Geometry check sheet. Reference: the model listing, model coordinates, mm. A direction names the side the tool comes from. Give positions to 0.01 mm unless a question says otherwise; leave off trailing zeros. Loops run counter-clockwise (first coordinate to the right, second up) from the corner with the lowest first, then second, coordinate; pieces in that order, holes last. Notation, with made-up numbers: (-32.75, -12.5) - (-15.75, -12.5) arc R22 cw to (-15.75, 3.5) - close; hole circle Ø3 at (-36, 86). An arc over 180 degrees is marked (long way). Use a Markdown table: item, result. Add a question column.
1. Cross-section at A-A on y = 3.75. Enter the section's corners in (x, z), and give its area (3 significant figures).
2. Draft check along Z on faces 4 (the flat face through (1, 5, 15.347)), 5 (the cylindrical face through (4.436, 12.686, 14.995)), 6 (the cylindrical face through (-16.435, 0.783, -11.827)), 7 (the flat face through (-18, 7, -4.453)). Enter one of: pulls with the +Z half, pulls with the -Z half, needs draft (parallel to the pull), parting line crosses it, or undercut.
3. Set-up check for faces 1 (the flat face through (-3.366, 7, 13)), 2 (the flat face through (6.134, 7, 13)), 3 (the flat face through (18, 7, -3.348)): record each of +Z, -Z, +X, -X, +Y, -Y from which the full face is reachable in a straight line by a thin tool's end or side.
4. Cross-section at B-B on z = 4. Enter the section's corners in (x, y), and give its area (3 significant figures).
5. Depth check by flat-ended pin: P1, Ø6, axis at y = 4.5, z = 12, coming from the +X side; P2, Ø3.5, axis at y = 8, z = 12.5, coming from the +X side; P3, Ø3.5, axis at y = 4.5, z = 12.5, coming from the -X side; P4, Ø10, axis at x = 1.5, z = 4.5, coming from the +Y side. Enter the tip coordinate at first touch or a pass-through.
6. Material ranges on L1, parallel to X at y = 4.5, z = 4.5; L2, parallel to Y at x = 0.5, z = 0; L3, parallel to Z at x = -15.5, y = 10, recorded low to high.
7. Cross-section at D-D on z = -12.5. Enter the section's corners in (x, y), and give its area (3 significant figures).
8. Cross-section at C-C on x = -18.5. Enter the section's corners in (y, z), and give its area (3 significant figures).
from build123d import *

# Parameters (mm, degrees)
SKETCH1_R           = 1.5875
BOSS_EXTRUDE4_DEPTH = 1.5875
SKETCH2_W           = 7.5057
SKETCH2_H           = 9.9695
BOSS_EXTRUDE5_DEPTH = 10.0711
SKETCH3_W           = 9.4996
SKETCH3_H           = 4.3434
BOSS_EXTRUDE6_DEPTH = 10.0965
SKETCH5_R           = 1.1303
BOSS_EXTRUDE7_DEPTH = 2.032
SKETCH6_W           = 7.5438
SKETCH6_H           = 9.9822
BOSS_EXTRUDE8_DEPTH = 11.1125


with BuildPart() as part:
    # Sketch1 → Boss-Extrude4 (new body)
    with BuildSketch(Plane(origin=(0, 0, 0), x_dir=(1, 0, 0), z_dir=(0, 1, 0))):
        with BuildLine():
            Line((21.881838929, -14.076705181), (21.881838929, 13.888694819))
            ThreePointArc((21.881838929, 13.888694819), (21.509864541, 14.786720431), (20.611838929, 15.158694819))
            Line((20.611838929, 15.158694819), (-20.612361071, 15.158694819))
            ThreePointArc((-20.612361071, 15.158694819), (-21.510386683, 14.786720431), (-21.882361071, 13.888694819))
            Line((-21.882361071, 13.888694819), (-21.882361071, -14.076705181))
            ThreePointArc((-21.882361071, -14.076705181), (-21.510386683, -14.974730793), (-20.612361071, -15.346705181))
            Line((-20.612361071, -15.346705181), (20.611838929, -15.346705181))
            ThreePointArc((20.611838929, -15.346705181), (21.509864541, -14.974730793), (21.881838929, -14.076705181))
        make_face()
        with Locations(Location((18.0086, 11.6205, 0), (0, 0, 270))):
            Circle(SKETCH1_R, mode=Mode.SUBTRACT)
        with Locations(Location((-18.0086, 11.6205, 0), (0, 0, 270))):
            Circle(SKETCH1_R, mode=Mode.SUBTRACT)
        with Locations(Location((-18.0086, -11.6205, 0), (0, 0, 270))):
            Circle(SKETCH1_R, mode=Mode.SUBTRACT)
        with Locations(Location((18.0086, -11.6205, 0), (0, 0, 270))):
            Circle(SKETCH1_R, mode=Mode.SUBTRACT)
    extrude(amount=BOSS_EXTRUDE4_DEPTH)

    # Sketch2 → Boss-Extrude5 (add)
    with BuildSketch(Plane(origin=(0, 1.5875, 0), x_dir=(1, 0, 0), z_dir=(0, 1, 0))):
        with Locations((18.128988929, -1.637055181)):
            Rectangle(SKETCH2_W, SKETCH2_H)
    extrude(amount=BOSS_EXTRUDE5_DEPTH)

    # Sketch3 → Boss-Extrude6 (add)
    with BuildSketch(Plane(origin=(0, 1.5875, 0), x_dir=(1, 0, 0), z_dir=(0, 1, 0))):
        with Locations((1.384038929, -13.175005181)):
            Rectangle(SKETCH3_W, SKETCH3_H)
    extrude(amount=BOSS_EXTRUDE6_DEPTH)

    # Sketch5 → Boss-Extrude7 (add)
    with BuildSketch(Plane(origin=(0, 11.684, 0), x_dir=(1, 0, 0), z_dir=(0, 1, 0))):
        with Locations(Location((4.485703039, -13.865914998, 0), (0, 0, 90))):
            Circle(SKETCH5_R)
    extrude(amount=BOSS_EXTRUDE7_DEPTH)

    # Sketch6 → Boss-Extrude8 (add)
    with BuildSketch(Plane(origin=(0, 1.5875, 0), x_dir=(1, 0, 0), z_dir=(0, 1, 0))):
        with Locations((-18.110461071, -0.538505181)):
            Rectangle(SKETCH6_W, SKETCH6_H)
    extrude(amount=BOSS_EXTRUDE8_DEPTH)


solid = part.part
Values found:
| question | item | result |
|---|---|---|
| 1 | outline | (-21.88, -4.45) - (-14.34, -4.45) - (-14.34, 5.53) - (-21.88, 5.53) - close; (-3.37, 11) - (6.13, 11) - (6.13, 15.35) - (-3.37, 15.35) - close; (14.38, -3.35) - (21.88, -3.35) - (21.88, 6.62) - (14.38, 6.62) - close |
| 1 | area | 191 mm2 |
| 2 | face 4 | pulls with the +Z half |
| 2 | face 5 | parting line crosses it |
| 2 | face 6 | undercut |
| 2 | face 7 | pulls with the -Z half |
| 3 | face 1 | +Z, -Z, -X, +Y |
| 3 | face 2 | +Z, -Z, +X, +Y |
| 3 | face 3 | -Z, +X, +Y |
| 4 | outline | (-21.88, 0) - (21.88, 0) - (21.88, 11.66) - (14.38, 11.66) - (14.38, 1.59) - (-14.34, 1.59) - (-14.34, 12.7) - (-21.88, 12.7) - close |
| 4 | area | 229 mm2 |
| 5 | P1 | stops at x = 21.88 |
| 5 | P2 | stops at x = 6.13 |
| 5 | P3 | stops at x = -3.37 |
| 5 | P4 | stops at y = 1.59 |
| 6 | L1 | x = -21.88 to -14.34, 14.38 to 21.88 |
| 6 | L2 | y = 0 to 1.59 |
| 6 | L3 | z = -4.45 to 5.53 |
| 7 | outline | (-21.88, 0) - (-19.33, 0) - (-19.33, 1.59) - (-21.88, 1.59) - close; (-16.69, 0) - (16.69, 0) - (16.69, 1.59) - (-16.69, 1.59) - close; (19.33, 0) - (21.88, 0) - (21.88, 1.59) - (19.33, 1.59) - close |
| 7 | area | 61.1 mm2 |
| 8 | outline | (0, -15.16) - (1.59, -15.16) - (1.59, -13.13) - (0, -13.13) - close; (0, -10.11) - (1.59, -10.11) - (1.59, -4.45) - (12.7, -4.45) - (12.7, 5.53) - (1.59, 5.53) - (1.59, 10.11) - (0, 10.11) - close; (0, 13.13) - (1.59, 13.13) - (1.59, 15.35) - (0, 15.35) - close |
| 8 | area | 150 mm2 |
